Work out the finished part from the listing and answer in its coordinate system (mm). Give positions to 0.01 mm unless a question says otherwise; leave off trailing zeros. Order: outer loops, then holes, each group sorted by start corner. A loop starts at its lowest first (then second) coordinate and runs counter-clockwise, first axis right, second up. Notation, with made-up numbers: M 23.25,22 L 67.25,22 A3 cw 67.25,27 Z; hole C -7.75,82 d1. An arc over 180 degrees is marked long. One line per item, written item: value.
from build123d import *

# Parameters (mm, degrees)
F0_R     = 7.07
F1_DEPTH = 10


with BuildPart() as f1:
    # F0 (on Right) → F1 (new body)
    with BuildSketch(Plane.YZ):
        with BuildLine():
            Line((0, 60), (0, 0))
            Line((0, 0), (35.842331, 18.949336))
            ThreePointArc((35.842331, 18.949336), (42.5, 30), (35.842331, 41.050664))
            Line((35.842331, 41.050664), (0, 60))
        make_face()
        with Locations((30, 30)):
            Circle(F0_R, mode=Mode.SUBTRACT)
    extrude(amount=F1_DEPTH)


solid = f1.part
(1) Section B-B, the plane y = 33 is taken. Give the vertices of the cut face in (x, z), then the cut area to 3 significant figures.
Findings:
outline: M 0,17.45 L 10,17.45 L 10,23.6 L 0,23.6 Z; M 0,36.4 L 10,36.4 L 10,42.55 L 0,42.55 Z
area: 123 mm^2
(2) Section A-A, the plane z = 30 is taken. Give the vertices of the cut face in (x, y), then the cut area to 3 significant figures.
Findings:
outline: M 0,0 L 10,0 L 10,22.93 L 0,22.93 Z; M 0,37.07 L 10,37.07 L 10,42.5 L 0,42.5 Z
area: 284 mm^2
(3) Determine the mould class of faces 1 (the cylindrical face through (4.9, 42.5, 29.8)), 2 (the flat face through (0, 16, 30)), 3 (the flat face through (5, 0, 30)), 4 (the cylindrical face through (4.93, 28.467, 23.098)) for opening direction Y: pulls with the +Y half, pulls with the -Y half, needs draft (parallel to the pull), parting line crosses it, or undercut.
Findings:
face 1: pulls with the +Y half
face 2: needs draft
face 3: pulls with the -Y half
face 4: undercut
(4) Section D-D, the plane z = 47 is taken. Give the vertices of the cut face in (x, y), then the cut area to 3 significant figures.
Findings:
outline: M 0,0 L 10,0 L 10,24.59 L 0,24.59 Z
area: 246 mm^2
(5) Section C-C, the plane x = 6 is taken. Give the vertices of the cut face in (y, z), then the cut area to 3 significant figures.
Findings:
outline: M 0,0 L 35.84,18.95 A12.5 ccw 35.84,41.05 L 0,60 Z; hole C 30,30 d14.14
area: 1,420 mm^2
(6) Find the intervals of material crossed by probe 1 along Z at (x, y) = (5, 32); probe 2 along Z at (x, y) = (2.5, 30); probe 3 along Y at (x, z) = (8.75, 32), in increasing order. Write a range as from..to.
Findings:
probe 1: z = 16.92..23.22, 36.78..43.08
probe 2: z = 15.86..22.93, 37.07..44.14
probe 3: y = 0..23.22, 36.78..42.34
(7) Given P1, Ø8.5, axis at y = 30, z = 30, coming from the -X side; P2, Ø5, axis at x = 5.5, z = 49, coming from the +Y side (3 decimals); P3, Ø6, axis at x = 3, z = 9.5, coming from the -Y side; P4, Ø3, axis at x = 8.5, y = 9, coming from the +Z side, each flat-ended and moving along its own axis, determine where each tip first touches the part or whether it passes through.
Findings:
P1: passes through
P2: stops at y = 25.535
P3: stops at y = 0
P4: stops at z = 56.03
